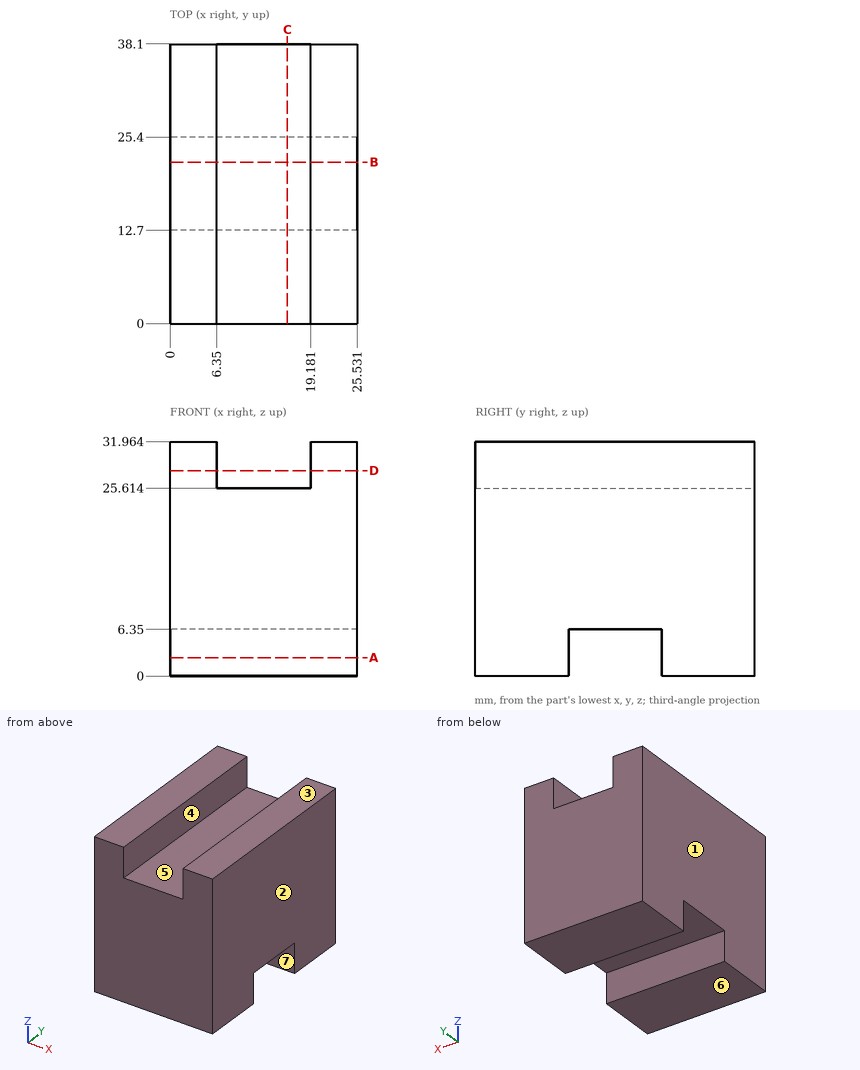
Print and shaded views of the part. All mm, measured from the part's lowest x, y and z. A direction names the side the tool comes from. Give positions to 0.01 mm unless a question says otherwise; leave off trailing zeros. Write each loop counter-clockwise with the first axis right and the second up, starting at its lowest first coordinate (ties: lowest second). Pieces come first, ordered by that corner, then holes. Notation, with made-up numbers: M 43,-39.75 L 84,-39.75 A27 ccw 84,-7.75 Z; hole C 48,79.25 d6. An arc over 180 degrees is marked long. Use a Markdown table: item, result.
1) Cut at C-C (x = 16). List the corners of the cut face in (y, z), and give its area (3 significant figures).
Responses:
| item | result |
|---|---|
| outline | M 0,0 L 12.7,0 L 12.7,6.35 L 25.4,6.35 L 25.4,0 L 38.1,0 L 38.1,25.61 L 0,25.61 Z |
| area | 895 mm2 |
2) Cut at B-B (y = 22). List the corners of the cut face in (x, z).
Responses:
| item | result |
|---|---|
| outline | M 0,6.35 L 25.53,6.35 L 25.53,31.96 L 19.18,31.96 L 19.18,25.61 L 6.35,25.61 L 6.35,31.96 L 0,31.96 Z |
3) Pin check, flat tips, straight feed: pin 1 (4 mm diameter, centred on x = 19, y = 17, fed in from -Z); pin 2 (1.5 mm diameter, centred on x = 18, y = 16, fed in from +Z). Stop position of each tip, or through.
Responses:
| item | result |
|---|---|
| pin 1 | stops at z = 6.35 |
| pin 2 | stops at z = 25.61 |
4) Pull direction X, two halves, no side cores. Call the marked faces 1, 2, 3 and 4: +X half, -X half, draft (parallel to the pull), parting line (faces both ways), or undercut.
Responses:
| item | result |
|---|---|
| face 1 | -X half |
| face 2 | +X half |
| face 3 | draft |
| face 4 | undercut |
5) Tool access for the marked faces 5, 6 and 7: list every direction of +Z, -Z, +X, -X, +Y, -Y with a clear straight run to the whole face (end or side of a thin tool).
Responses:
| item | result |
|---|---|
| face 5 | +Z, +Y, -Y |
| face 6 | -Z, +X, -X, +Y, -Y |
| face 7 | -Z, +X, -X |
6) Cut at A-A (z = 2.5). List the corners of the cut face in (x, y).
Responses:
| item | result |
|---|---|
| outline | M 0,0 L 25.53,0 L 25.53,12.7 L 0,12.7 Z; M 0,25.4 L 25.53,25.4 L 25.53,38.1 L 0,38.1 Z |
7) Drill centre lines: line 1 (Y direction, x = 22.25, z = 6); line 2 (X direction, y = 35, z = 30.5); line 3 (Z direction, x = 10.5, y = 14). Where is each one in solid material? Low to high. Write a range as from..to.
Responses:
| item | result |
|---|---|
| line 1 | y = 0..12.7, 25.4..38.1 |
| line 2 | x = 0..6.35, 19.18..25.53 |
| line 3 | z = 6.35..25.61 |
8) Cut at D-D (z = 28). List the corners of the cut face in (x, y).
Responses:
| item | result |
|---|---|
| outline | M 0,0 L 6.35,0 L 6.35,38.1 L 0,38.1 Z; M 19.18,0 L 25.53,0 L 25.53,38.1 L 19.18,38.1 Z |
